from build123d import *

# Parameters (mm, degrees)
SKETCH2_R           = 2
SKETCH2_R_2         = 2.5
BOSS_EXTRUDE1_DEPTH = 10
SKETCH3_R           = 10
BOSS_EXTRUDE3_DEPTH = 20
CUT_EXTRUDE1_REACH  = 22
SKETCH4_R           = 7.75


with BuildPart() as part:
    # Sketch2 → Boss-Extrude1 (new body)
    with BuildSketch(Plane(origin=(0, 0, 0), x_dir=(1, 0, 0), z_dir=(0, 1, 0))):
        with BuildLine():
            Line((0, 7.5), (100, 7.5))
            ThreePointArc((100, 7.5), (107.5, 0), (100, -7.5))
            Line((100, -7.5), (0, -7.5))
            ThreePointArc((0, -7.5), (-7.5, 0), (0, 7.5))
        make_face()
        Circle(SKETCH2_R, mode=Mode.SUBTRACT)
        with Locations((100, 0)):
            Circle(SKETCH2_R_2, mode=Mode.SUBTRACT)
    extrude(amount=BOSS_EXTRUDE1_DEPTH)

    # Sketch3 → Boss-Extrude3 (add)
    with BuildSketch(Plane(origin=(0, 0, 0), x_dir=(1, 0, 0), z_dir=(0, 1, 0))):
        with Locations((100, 0)):
            Circle(SKETCH3_R)
    extrude(amount=BOSS_EXTRUDE3_DEPTH)

    # Sketch4 → Cut-Extrude1 (cut, up to next)
    with BuildSketch(Plane(origin=(0, 20, 0), x_dir=(1, 0, 0), z_dir=(0, 1, 0)), mode=Mode.PRIVATE) as cut_extrude1_sk1:
        with Locations((100, 0)):
            Circle(SKETCH4_R)
    cut_extrude1_tool1 = extrude(cut_extrude1_sk1.sketch, amount=-CUT_EXTRUDE1_REACH, mode=Mode.PRIVATE) & part.part
    add(cut_extrude1_tool1.solids().sort_by_distance((100, 20, 0))[0], mode=Mode.SUBTRACT)


solid = part.part
The model under review builds one solid part; all positions refer to its coordinate system, in mm. A direction names the side the tool comes from. Round coordinates to 2 decimals unless told otherwise and drop trailing zeros. Order: outer loops, then holes, each group sorted by start corner. A loop starts at its lowest first (then second) coordinate and runs counter-clockwise, first axis right, second up. Notation, with made-up numbers: (-37, 16.25) -> (10, 16.25) arc R16 ccw to (10, 39.25) -> close; hole circle Ø8 at (-20, -3.75). An arc over 180 degrees is marked (long way). Write item = value, one per line. Start each with the question number.
Item 1: Clearance check with flat-ended pins moving along their axes: pin 1 Ø1 at (x, y) = (29, 8) entering from +Z; pin 2 Ø1 at (y, z) = (6.5, -8) entering from +X; pin 3 Ø4 at (x, y) = (93, 4) entering from -Z. State where each tip first meets the part, or that it passes through.
Item 2: For line 1 along X through (y, z) = (7.5, 0); line 2 along Z through (x, y) = (100, 15.75); line 3 along Y through (x, z) = (57, 6.75), list the stretches that pass through material, from the lowest coordinate up.
Item 3: Consider section A-A on x = 100. Write out the cut boundary in (y, z), plus the area to 3 significant figures.
Item 4: Consider section D-D on y = 14. Write out the cut boundary in (x, z).
Item 5: Mouldability with a two-part tool opening along X and no side actions: class faces 3 (the face through (0, 5, 2)), 4 (the face through (47, 5, 7.5)), 5 (the face through (109.237, 9.86, 3.83)) as released by +X, released by -X, zero draft, split by the parting line, or undercut.
Item 6: Consider section B-B on y = 2.75. Write out the cut boundary in (x, z).
Item 7: Consider section C-C on z = -5.5. Write out the cut boundary in (x, y).
Item 8: For faces 1 (the face through (46, 5, -7.5)), 2 (the face through (102.9, 20, 7.4)), list the 3-axis set-ups (+Z, -Z, +X, -X, +Y, -Y) from which the entire face can be reached by the end or side of a thin tool; tool diameter is ignored.
Conclusion:
q1.pin_1 = 7.5
q1.pin_2 = 106.61
q1.pin_3 = -8.66
q2.line_1 = -7.5 to -2, 2 to 92.25, 107.75 to 110
q2.line_2 = -10 to -7.75, 7.75 to 10
q2.line_3 = 0 to 10
q3.outline = (0, -10) -> (20, -10) -> (20, -7.75) -> (0, -7.75) -> close; (0, 7.75) -> (20, 7.75) -> (20, 10) -> (0, 10) -> close
q3.area = 90.0 mm2
q4.outline = circle Ø20 at (100, 0); hole circle Ø15.5 at (100, 0)
q5.face_3 = undercut
q5.face_4 = zero draft
q5.face_5 = split by the parting line
q6.outline = (0, -7.5) -> (93.39, -7.5) arc R10 ccw (long way) to (93.39, 7.5) -> (0, 7.5) arc R7.5 ccw to start; hole circle Ø4 at (0, 0); hole circle Ø15.5 at (100, 0)
q7.outline = (-5.1, 0) -> (94.54, 0) -> (94.54, 20) -> (91.65, 20) -> (91.65, 10) -> (-5.1, 10) -> close; (105.46, 0) -> (108.35, 0) -> (108.35, 20) -> (105.46, 20) -> close
q8.face_1 = -Z, -X, +Y, -Y
q8.face_2 = +Z, -Z, +X, -X, +Y
